```python
from build123d import *

# Parameters (mm, degrees)
DODANIE_WYCI_GNI_CIE1_DEPTH = 400


with BuildPart() as part:
    # Szkic1 → Dodanie-wyciągnięcie1 (new body)
    with BuildSketch(Plane.XY):
        with BuildLine():
            Line((4.385786438, 5.8), (0, 5.8))
            Line((0, 5.8), (-4.385786438, 5.8))
            Line((-4.385786438, 5.8), (-8.5, 9.914213562))
            Line((-8.5, 9.914213562), (-8.5, 13.5))
            Line((-8.5, 13.5), (-4, 13.5))
            Line((-4, 13.5), (-4, 15))
            Line((-4, 15), (-13, 15))
            ThreePointArc((-13, 15), (-14.414213562, 14.414213562), (-15, 13))
            Line((-15, 13), (-15, 4))
            Line((-15, 4), (-13.5, 4))
            Line((-13.5, 4), (-13.5, 8.5))
            Line((-13.5, 8.5), (-9.914213562, 8.5))
            Line((-9.914213562, 8.5), (-5.8, 4.385786438))
            Line((-5.8, 4.385786438), (-5.8, 0))
            Line((-5.8, 0), (-5.8, -4.385786438))
            Line((-5.8, -4.385786438), (-9.914213562, -8.5))
            Line((-9.914213562, -8.5), (-13.5, -8.5))
            Line((-13.5, -8.5), (-13.5, -4))
            Line((-13.5, -4), (-15, -4))
            Line((-15, -4), (-15, -13))
            ThreePointArc((-15, -13), (-14.414213562, -14.414213562), (-13, -15))
            Line((-13, -15), (-4, -15))
            Line((-4, -15), (-4, -13.5))
            Line((-4, -13.5), (-8.5, -13.5))
            Line((-8.5, -13.5), (-8.5, -9.914213562))
            Line((-8.5, -9.914213562), (-4.385786438, -5.8))
            Line((-4.385786438, -5.8), (0, -5.8))
            Line((0, -5.8), (4.385786438, -5.8))
            Line((4.385786438, -5.8), (8.5, -9.914213562))
            Line((8.5, -9.914213562), (8.5, -13.5))
            Line((8.5, -13.5), (4, -13.5))
            Line((4, -13.5), (4, -15))
            Line((4, -15), (13, -15))
            ThreePointArc((13, -15), (14.414213562, -14.414213562), (15, -13))
            Line((15, -13), (15, -4))
            Line((15, -4), (13.5, -4))
            Line((13.5, -4), (13.5, -8.5))
            Line((13.5, -8.5), (9.914213562, -8.5))
            Line((9.914213562, -8.5), (5.8, -4.385786438))
            Line((5.8, -4.385786438), (5.8, 0))
            Line((5.8, 0), (5.8, 4.385786438))
            Line((5.8, 4.385786438), (9.914213562, 8.5))
            Line((9.914213562, 8.5), (13.5, 8.5))
            Line((13.5, 8.5), (13.5, 4))
            Line((13.5, 4), (15, 4))
            Line((15, 4), (15, 13))
            ThreePointArc((15, 13), (14.414213562, 14.414213562), (13, 15))
            Line((13, 15), (4, 15))
            Line((4, 15), (4, 13.5))
            Line((4, 13.5), (8.5, 13.5))
            Line((8.5, 13.5), (8.5, 9.914213562))
            Line((8.5, 9.914213562), (4.385786438, 5.8))
        make_face()
        with BuildLine():
            Line((-13.5, -10), (-10, -10))
            Line((-10, -10), (-10, -13.5))
            Line((-10, -13.5), (-13, -13.5))
            ThreePointArc((-13, -13.5), (-13.353553391, -13.353553391), (-13.5, -13))
            Line((-13.5, -13), (-13.5, -10))
        make_face(mode=Mode.SUBTRACT)
        with BuildLine():
            Line((10, -13.5), (10, -10))
            Line((10, -10), (13.5, -10))
            Line((13.5, -10), (13.5, -13))
            ThreePointArc((13.5, -13), (13.353553391, -13.353553391), (13, -13.5))
            Line((13, -13.5), (10, -13.5))
        make_face(mode=Mode.SUBTRACT)
        with BuildLine():
            ThreePointArc((3.4, 0), (2.404163056, -2.404163056), (0, -3.4))
            ThreePointArc((0, -3.4), (-2.404163056, -2.404163056), (-3.4, 0))
            ThreePointArc((-3.4, 0), (-2.404163056, 2.404163056), (0, 3.4))
            ThreePointArc((0, 3.4), (2.404163056, 2.404163056), (3.4, 0))
        make_face(mode=Mode.SUBTRACT)
        with BuildLine():
            Line((-10, 13.5), (-10, 10))
            Line((-10, 10), (-13.5, 10))
            Line((-13.5, 10), (-13.5, 13))
            ThreePointArc((-13.5, 13), (-13.353553391, 13.353553391), (-13, 13.5))
            Line((-13, 13.5), (-10, 13.5))
        make_face(mode=Mode.SUBTRACT)
        with BuildLine():
            Line((10, 10), (10, 13.5))
            Line((10, 13.5), (13, 13.5))
            ThreePointArc((13, 13.5), (13.353553391, 13.353553391), (13.5, 13))
            Line((13.5, 13), (13.5, 10))
            Line((13.5, 10), (10, 10))
        make_face(mode=Mode.SUBTRACT)
    extrude(amount=DODANIE_WYCI_GNI_CIE1_DEPTH)


solid = part.part
```
For this review, take the finished solid that the model builds, in its own axes (mm). Give positions to 0.01 mm unless a question says otherwise; leave off trailing zeros.
1) The part is to be moulded in two halves that separate along X. For faces 1 (the face through (15, -9, 197)), 2 (the face through (-8, 15, 197)), 3 (the face through (0, -5.8, 197)), say which applies: released by +X, released by -X, zero draft, split by the parting line, or undercut.
2) Wall thickness on line 1 (X direction, y = -13.25, z = 315); line 2 (X direction, y = 10.75, z = 172): over which ranges is each line inside the solid? List them lowest first.
3) Insertion check: pin 1 (1.2 mm diameter, centred on y = 14.5, z = 255.5, fed in from -X); pin 2 (7 mm diameter, centred on x = 0, z = 211, fed in from -Y). Each pin has a flat end and moves straight along its axis. Give the tip position at first contact, or say it passes through.
4) Take a section at A-A (z = 182.5). State how many separate pieces and enclosed holes the cut face has, then the cut area to 3 significant figures.
Derived:
1. face 1: released by +X
1. face 2: zero draft
1. face 3: undercut
2. line 1: x = -14.98 to -13.43, -10 to -8.5, 8.5 to 10, 13.43 to 14.98
2. line 2: x = -15 to -13.5, -10 to -8.5, 8.5 to 10, 13.5 to 15
3. pin 1: stops at x = -14.79
3. pin 2: stops at y = -5.8
4. separate pieces: 1
4. enclosed holes: 5
4. area: 308 mm2
